Read the model definition and answer for the solid it produces. Units are mm, in the model's axes. A direction names the side the tool comes from. Round coordinates to 2 decimals unless told otherwise and drop trailing zeros. Write each loop counter-clockwise with the first axis right and the second up, starting at its lowest first coordinate (ties: lowest second). Pieces come first, ordered by that corner, then holes. Notation, with made-up numbers: (37.5, 69.5) - (51.5, 69.5) arc R17 cw to (51.5, 102.5) - close; hole circle Ø5 at (4.25, 10). An arc over 180 degrees is marked (long way). One line per item, written item: value. Start each with the question number.
(1) Flat-ended cylindrical pins translate along their axes: pin 1 Ø5 at (x, y) = (7.5, -27) entering from +Z; pin 2 Ø12 at (x, z) = (-44.5, 25.5) entering from -Y; pin 3 Ø4 at (x, z) = (-51.5, 29) entering from -Y; pin 4 Ø5 at (x, y) = (-22, -6) entering from -Z. Find the tip coordinate at first contact, or state that the pin passes through.
(2) Find the intervals of material crossed by L1, parallel to Y at x = 0, z = 45.5; L2, parallel to Z at x = 28, y = 19.5; L3, parallel to Z at x = -25, y = 60, in increasing order.
(3) A cutting plane is placed at B-B, the plane z = 39. Determine the outline of the cut face in (x, y).
(4) For faces 1 (the face through (-1, 1, 2)), 2 (the face through (-16, -4, 0)), 3 (the face through (-1.73, -7.81, 37.35)), determine the directions among +Z, -Z, +X, -X, +Y, -Y from which every point of the face is accessible in a straight line to the end or side of a thin tool.
(5) A cutting plane is placed at A-A, the plane x = 0. Determine the outline of the cut face in (y, z), plus the area to 3 significant figures.
(6) The mould has two halves that part along Y. Classify faces 4 (the face through (-17.34, -78.1, 32.82)), 5 (the face through (-28.211, -15.638, 0.986)), 6 (the face through (-15, -67, 10)): +Y half, -Y half, draft (parallel to the pull), parting line (faces both ways), or undercut.
from build123d import *

# Parameters (mm, degrees)
SKETCH1_R           = 80
BOSS_EXTRUDE1_DEPTH = 62
SKETCH3_OUTSIDE_W   = 228.922
SKETCH3_OUTSIDE_H   = 228.922
SKETCH3_OUTSIDE_R   = 54
CUT_EXTRUDE1_DEPTH  = 10
CUT_EXTRUDE1_DRAFT  = -45
SKETCH4_OUTSIDE_W   = 213.586
SKETCH4_OUTSIDE_H   = 213.586
SKETCH4_OUTSIDE_R   = 20
CUT_EXTRUDE2_DEPTH  = 5
CUT_EXTRUDE2_DRAFT  = -25
CUT_EXTRUDE3_DEPTH  = 2
SKETCH6_OUTSIDE_W   = 209.028
SKETCH6_OUTSIDE_H   = 209.028
SKETCH6_OUTSIDE_R   = 70
CUT_EXTRUDE4_DEPTH  = 1
CUT_EXTRUDE4_DRAFT  = -3
SKETCH2_R           = 8
CUT_EXTRUDE5_DEPTH  = 50


with BuildPart() as part:
    # Sketch1 → Boss-Extrude1 (new body)
    with BuildSketch(Plane.XY):
        Circle(SKETCH1_R)
    extrude(amount=BOSS_EXTRUDE1_DEPTH)


with BuildPart() as cut_extrude1_tool:
    # Sketch3 outside → Cut-Extrude1 (with draft: the straight prism first)
    with BuildSketch(Plane(origin=(0, 0, 0), x_dir=(-1, 0, 0), z_dir=(0, 0, -1))):
        Rectangle(SKETCH3_OUTSIDE_W, SKETCH3_OUTSIDE_H)
        Circle(SKETCH3_OUTSIDE_R, mode=Mode.SUBTRACT)
    extrude(amount=-CUT_EXTRUDE1_DEPTH)
    # Cut-Extrude1: the draft: its side faces are tilted about the plane it starts from
    cut_extrude1_sides = [cut_extrude1_tool.faces().sort_by_distance(p)[0] for p in [
        (0, -114.461, 5),
        (-114.461, 0, 5),
        (0, 114.461, 5),
        (114.461, 0, 5),
        (54, 0, 5),
    ]]
    draft(cut_extrude1_sides, Plane(origin=(0, 0, 0), x_dir=(-1, 0, 0), z_dir=(0, 0, -1)), CUT_EXTRUDE1_DRAFT)


with BuildPart() as part_1:
    add(part.part)

    # Cut-Extrude1: cut by cut_extrude1_tool
    add(cut_extrude1_tool.part, mode=Mode.SUBTRACT)


with BuildPart() as cut_extrude2_tool:
    # Sketch4 outside → Cut-Extrude2 (with draft: the straight prism first)
    with BuildSketch(Plane.XY.offset(62)):
        Rectangle(SKETCH4_OUTSIDE_W, SKETCH4_OUTSIDE_H)
        Circle(SKETCH4_OUTSIDE_R, mode=Mode.SUBTRACT)
    extrude(amount=-CUT_EXTRUDE2_DEPTH)
    # Cut-Extrude2: the draft: its side faces are tilted about the plane it starts from
    cut_extrude2_sides = [cut_extrude2_tool.faces().sort_by_distance(p)[0] for p in [
        (0, -106.793, 59.5),
        (106.793, 0, 59.5),
        (0, 106.793, 59.5),
        (-106.793, 0, 59.5),
        (-20, 0, 59.5),
    ]]
    draft(cut_extrude2_sides, Plane.XY.offset(62), CUT_EXTRUDE2_DRAFT)


with BuildPart() as part_2:
    add(part_1.part)

    # Cut-Extrude2: cut by cut_extrude2_tool
    add(cut_extrude2_tool.part, mode=Mode.SUBTRACT)

    # Sketch5 → Cut-Extrude3 (cut)
    with BuildSketch(Plane(origin=(0, 0, 0), x_dir=(-1, 0, 0), z_dir=(0, 0, -1))):
        with BuildLine():
            Line((10.970305524, 10.229975401), (36.567685081, 34.099918003))
            ThreePointArc((36.567685081, 34.099918003), (47.552825815, 15.450849719), (49.627307582, -6.09346717))
            Line((49.627307582, -6.09346717), (14.888192275, -1.828040151))
            ThreePointArc((14.888192275, -1.828040151), (14.265847744, -4.635254916), (13.119295607, -7.272144304))
            Line((13.119295607, -7.272144304), (43.730985357, -24.240481012))
            ThreePointArc((43.730985357, -24.240481012), (29.389262615, -40.450849719), (9.540449769, -49.081359172))
            Line((9.540449769, -49.081359172), (2.862134931, -14.724407752))
            ThreePointArc((2.862134931, -14.724407752), (0, -15), (-2.862134931, -14.724407752))
            Line((-2.862134931, -14.724407752), (-9.540449769, -49.081359172))
            ThreePointArc((-9.540449769, -49.081359172), (-29.389262615, -40.450849719), (-43.730985357, -24.240481012))
            Line((-43.730985357, -24.240481012), (-13.119295607, -7.272144304))
            ThreePointArc((-13.119295607, -7.272144304), (-14.265847744, -4.635254916), (-14.888192275, -1.828040151))
            Line((-14.888192275, -1.828040151), (-49.627307582, -6.09346717))
            ThreePointArc((-49.627307582, -6.09346717), (-47.552825815, 15.450849719), (-36.567685081, 34.099918003))
            Line((-36.567685081, 34.099918003), (-10.970305524, 10.229975401))
            ThreePointArc((-10.970305524, 10.229975401), (-8.816778784, 12.135254916), (-6.339273926, 13.594616806))
            Line((-6.339273926, 13.594616806), (-21.130913087, 45.315389352))
            ThreePointArc((-21.130913087, 45.315389352), (0, 50), (21.130913087, 45.315389352))
            Line((21.130913087, 45.315389352), (6.339273926, 13.594616806))
            ThreePointArc((6.339273926, 13.594616806), (8.816778784, 12.135254916), (10.970305524, 10.229975401))
        make_face()
    extrude(amount=-CUT_EXTRUDE3_DEPTH, mode=Mode.SUBTRACT)


with BuildPart() as cut_extrude4_tool:
    # Sketch6 outside → Cut-Extrude4 (with draft: the straight prism first)
    with BuildSketch(Plane.XY.offset(57)):
        Rectangle(SKETCH6_OUTSIDE_W, SKETCH6_OUTSIDE_H)
        Circle(SKETCH6_OUTSIDE_R, mode=Mode.SUBTRACT)
    extrude(amount=-CUT_EXTRUDE4_DEPTH)
    # Cut-Extrude4: the draft: its side faces are tilted about the plane it starts from
    cut_extrude4_sides = [cut_extrude4_tool.faces().sort_by_distance(p)[0] for p in [
        (0, -104.514, 56.5),
        (104.514, 0, 56.5),
        (0, 104.514, 56.5),
        (-104.514, 0, 56.5),
        (-70, 0, 56.5),
    ]]
    draft(cut_extrude4_sides, Plane.XY.offset(57), CUT_EXTRUDE4_DRAFT)


with BuildPart() as part_3:
    add(part_2.part)

    # Cut-Extrude4: cut by cut_extrude4_tool
    add(cut_extrude4_tool.part, mode=Mode.SUBTRACT)

    # Fillet1: read off the stored shape, not the designer's step
    # Fillet1 outline → Fillet1 (revolve, cut)
    with BuildSketch(Plane.XZ):
        with BuildLine():
            ThreePointArc((80, 20), (77.071067812, 12.928932188), (70, 10))
            Line((70, 10), (80, 10))
            Line((80, 10), (80, 20))
        make_face()
        with BuildLine():
            ThreePointArc((70.052407779, 56), (77.089572547, 53.052651853), (80, 46.00013733))
            Line((80, 46.00013733), (80, 56))
            Line((80, 56), (70.052407779, 56))
        make_face()
    revolve(axis=Axis((0, 0, 0), (0, 0, 1)), mode=Mode.SUBTRACT)

    # Fillet1 2 outline → Fillet1 2 (revolve)
    with BuildSketch(Plane.XZ):
        with BuildLine():
            Line((61.071067812, 10), (61.071067812, 7.071067812))
            ThreePointArc((61.071067812, 7.071067812), (64.3153013, 9.238795325), (68.142135624, 10))
            Line((68.142135624, 10), (61.071067812, 10))
        make_face()
    revolve(axis=Axis((0, 0, 0), (0, 0, 1)))

    # Sketch2 → Cut-Extrude5 (cut)
    with BuildSketch(Plane.XY.offset(62)):
        Circle(SKETCH2_R)
    extrude(amount=-CUT_EXTRUDE5_DEPTH, mode=Mode.SUBTRACT)


solid = part_3.part
Here are the results:
1. pin 1: z = 57
1. pin 2: y = -70.13
1. pin 3: y = -62.85
1. pin 4: z = 0
2. L1: -80 to -8, 8 to 80
2. L2: 2 to 57
2. L3: 9.49 to 57
3. outline: circle Ø160 at (0, 0); hole circle Ø16 at (0, 0)
4. face 1: -Z
4. face 2: -Z, +X, -X, +Y, -Y
4. face 3: +Z
5. outline: (-80, 20) arc R10 ccw to (-70, 10) - (-68.14, 10) arc R10 cw to (-61.07, 7.07) - (-54, 0) - (-15, 0) - (-15, 2) - (50, 2) - (50, 0) - (54, 0) - (61.07, 7.07) arc R10 cw to (68.14, 10) - (70, 10) arc R10 ccw to (80, 20) - (80, 46) arc R10 ccw to (70.05, 56) - (70, 57) - (22.33, 57) - (20, 62) - (8, 62) - (8, 12) - (-8, 12) - (-8, 62) - (-20, 62) - (-22.33, 57) - (-70, 57) - (-70.05, 56) arc R10 ccw to (-80, 46) - close
5. area: 7,880 mm²
6. face 4: parting line
6. face 5: undercut
6. face 6: draft
